Answer from the drawing. Dimensions are ordinates in mm from the lowest x, y and z of the part. Give positions to 0.01 mm unless a question says otherwise; leave off trailing zeros. Order: outer loops, then holes, each group sorted by start corner. A loop starts at its lowest first (then second) coordinate and runs counter-clockwise, first axis right, second up. Notation, with made-up numbers: (-10.5, 13) - (25.5, 13) arc R15 ccw to (25.5, 32) - close; hole circle Ø2 at (81.5, 1.25). An arc over 180 degrees is marked (long way). Answer in a Markdown table with one row per item.
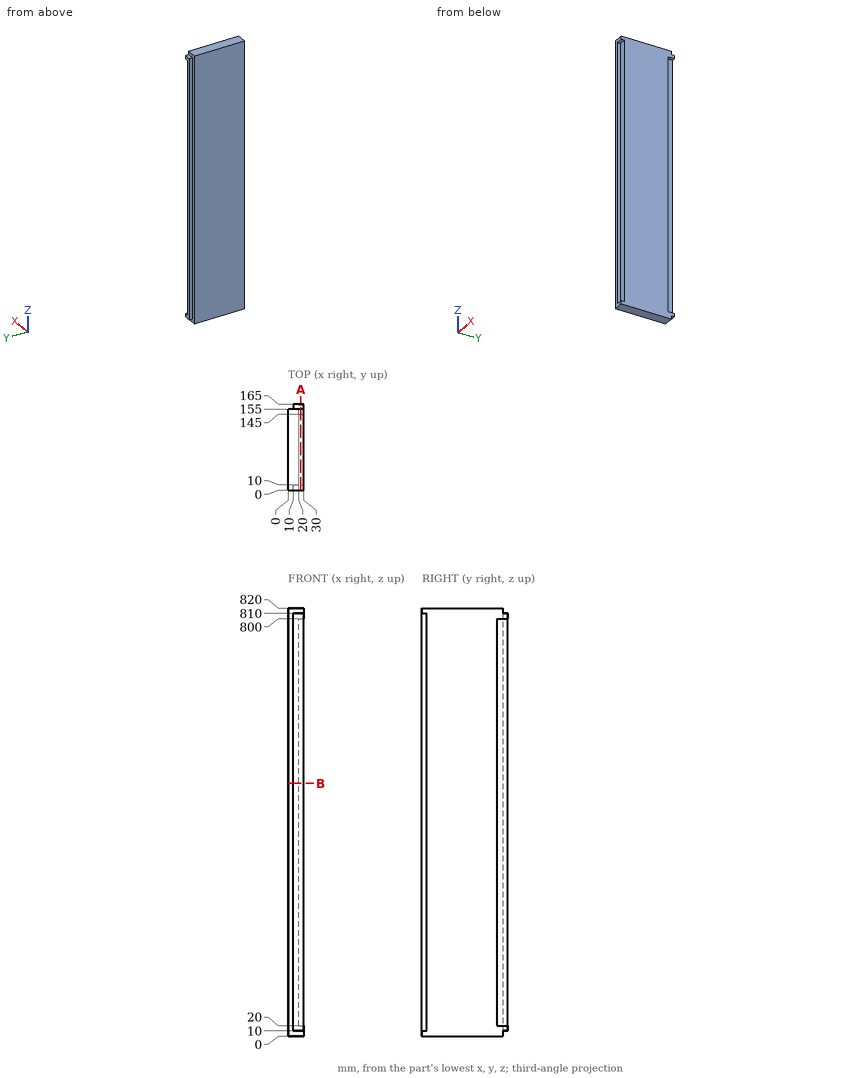
Item 1: Each of these flat-tipped pins is pushed along its axis until it touches: P1, Ø8, axis at y = 5, z = 452.5, coming from the +X side; P2, Ø10, axis at x = 18, z = 216, coming from the -Y side; P3, Ø8, axis at x = 22, y = 162.5, coming from the -Z side. Where does it stop, or does it pass through?
Answer block:
| item | result |
|---|---|
| P1 | x = 10 |
| P2 | y = 10 |
| P3 | z = 10 |
Item 2: Find section A-A on x = 24.5. Write down the section's boundary in (y, z).
Answer block:
| item | result |
|---|---|
| outline | (0, 0) - (155, 0) - (155, 10) - (165, 10) - (165, 20) - (145, 20) - (145, 800) - (165, 800) - (165, 810) - (155, 810) - (155, 820) - (0, 820) - (0, 810) - (10, 810) - (10, 10) - (0, 10) - close |
Item 3: Find section B-B on z = 484. Write down the section's boundary in (x, y).
Answer block:
| item | result |
|---|---|
| outline | (0, 0) - (10, 0) - (10, 10) - (30, 10) - (30, 145) - (20, 145) - (20, 165) - (10, 165) - (10, 155) - (0, 155) - close |
Item 4: Consider line 1 (Z direction, x = 13.25, y = 9); line 2 (Y direction, x = 27.25, z = 448.5); line 3 (Y direction, x = 16.5, z = 745.5). Determine where each line is inside the solid, lowest interval first.
Answer block:
| item | result |
|---|---|
| line 1 | 0 to 10, 810 to 820 |
| line 2 | 10 to 145 |
| line 3 | 10 to 165 |
